Geometry check sheet. Reference: the model listing, model coordinates, mm. A direction names the side the tool comes from. Round coordinates to 2 decimals unless told otherwise and drop trailing zeros. Loops run counter-clockwise (first coordinate to the right, second up) from the corner with the lowest first, then second, coordinate; pieces in that order, holes last. Notation, with made-up numbers: (8, -31.75) -> (21, -31.75) arc R9 ccw to (21, -23.75) -> close; hole circle Ø10 at (58, 12.5). An arc over 180 degrees is marked (long way). Use a Markdown table: item, result. Add a question column.
Q1. Material ranges on L1, parallel to X at y = 103, z = -11; L2, parallel to X at y = 62, z = -6; L3, parallel to Z at x = 36, y = 63, recorded low to high.
Q2. Gauge pin test, flat ends, axial feed: P1, Ø1.5, axis at y = 96, z = -16.5, coming from the -X side; P2, Ø3, axis at x = 73.5, y = 85.5, coming from the +Z side; P3, Ø1.6, axis at x = 75, y = 144, coming from the +Z side; P4, Ø4, axis at x = 3.175, z = 3.175, coming from the -Y side. Record the tip position at first contact, or that the pin passes through.
Q3. Release check for a two-part mould opening along Y. For faces 1 (the face through (35, 0, -15)), 2 (the face through (73, 12.7, -5)), 3 (the face through (69.85, 75, -9)) record: released by +Y, released by -Y, zero draft, split by the parting line, or undercut.
Q4. Sectioned sample at A-A, the plane y = 108.5. Enter the section's corners in (x, z), then the cut area to 3 significant figures.
Q5. Sectioned sample at B-B, the plane x = 44. Enter the section's corners in (y, z).
Q6. Set-up check for faces 4 (the face through (70.755, 6.439, -1.209)), 5 (the face through (73, 75, -6.604)), 6 (the face through (75, 6, -0.254)): record each of +Z, -Z, +X, -X, +Y, -Y from which the full face is reachable in a straight line by a thin tool's end or side.
```python
from build123d import *

# Parameters (mm, degrees)
F1_DEPTH  = 152.4
F2_R      = 5.08
F4_R      = 1.27
F5_DEPTH  = 76.201
F6_W      = 12.7
F6_H      = 6.35
F7_DEPTH  = 6.35
F8_W      = 12.7
F8_H      = 6.35
F9_DEPTH  = 6.35
F10_R     = 1.27
F11_DEPTH = 152.401
F12_R     = 3.175


with BuildPart() as f1:
    # F0 (on Front) → F1 (new body)
    with BuildSketch(Plane.XZ):
        Polygon((0, 0), (0, -19.558), (76.2, -19.558), (76.2, -6.604), (69.85, -6.604), (69.85, -13.208), (6.35, -13.208), (6.35, 0), align=None)
    extrude(amount=-F1_DEPTH)

    # F2
    f2_edges = [f1.edges().sort_by_distance(p)[0] for p in [
        (0, 76.2, -19.558),
        (76.2, 76.2, -19.558),
    ]]
    fillet(f2_edges, radius=F2_R)

    # F4 (on face) → F5 (cut, through all)
    with BuildSketch(Plane(origin=(0, 0, 0), x_dir=(0, -1, 0), z_dir=(-1, 0, 0))):
        with Locations((-149.225, -10.033)):
            Circle(F4_R)
        with Locations((-3.175, -10.033)):
            Circle(F4_R)
    extrude(amount=-F5_DEPTH, mode=Mode.SUBTRACT)

    # F6 (on face) → F7 (join)
    with BuildSketch(Plane.YZ.offset(76.2)):
        with Locations((6.35, -3.429)):
            Rectangle(F6_W, F6_H)
        with Locations((146.05, -3.429)):
            Rectangle(F6_W, F6_H)
    extrude(amount=-F7_DEPTH)

    # F8 (on face) → F9 (join)
    with BuildSketch(Plane(origin=(0, 0, 0), x_dir=(0, -1, 0), z_dir=(-1, 0, 0))):
        with Locations((-146.05, 3.175)):
            Rectangle(F8_W, F8_H)
        with Locations((-6.35, 3.175)):
            Rectangle(F8_W, F8_H)
    extrude(amount=-F9_DEPTH)

    # F10 (on face) → F11 (cut, through all)
    with BuildSketch(Plane.XZ):
        with Locations((73.025, -3.429)):
            Circle(F10_R)
        with Locations((3.175, 3.175)):
            Circle(F10_R)
    extrude(amount=-F11_DEPTH, mode=Mode.SUBTRACT)

    # F12
    f12_edges = [f1.edges().sort_by_distance(p)[0] for p in [
        (69.85, 6.35, -0.254),
        (69.85, 146.05, -0.254),
        (6.35, 6.35, 6.35),
        (6.35, 146.05, 6.35),
    ]]
    fillet(f12_edges, radius=F12_R)


solid = f1.part
```
Values:
| question | item | result |
|---|---|---|
| 1 | L1 | 0 to 6.35, 69.85 to 76.2 |
| 1 | L2 | 0 to 6.35 |
| 1 | L3 | -19.56 to -13.21 |
| 2 | P1 | x = 0.16 |
| 2 | P2 | z = -6.6 |
| 2 | P3 | z = -0.25 |
| 2 | P4 | y = 0 |
| 3 | face 1 | released by -Y |
| 3 | face 2 | undercut |
| 3 | face 3 | zero draft |
| 4 | outline | (0, -14.48) arc R5.08 ccw to (5.08, -19.56) -> (71.12, -19.56) arc R5.08 ccw to (76.2, -14.48) -> (76.2, -6.6) -> (69.85, -6.6) -> (69.85, -13.21) -> (6.35, -13.21) -> (6.35, 0) -> (0, 0) -> close |
| 4 | area | 599 mm^2 |
| 5 | outline | (0, -19.56) -> (152.4, -19.56) -> (152.4, -13.21) -> (0, -13.21) -> close |
| 6 | face 4 | +Z, +Y, -Y |
| 6 | face 5 | +Z, +X |
| 6 | face 6 | +Z, +X, +Y, -Y |
